```python
from build123d import *

# Parameters (mm, degrees)
SKETCH4_R          = 3
CUT_EXTRUDE1_DEPTH = 11


with BuildPart() as part:
    # Sweep2: sweep along a path in Sketch1
    with BuildLine(Plane(origin=(0, 0, 0), x_dir=(1, 0, 0), z_dir=(0, 1, 0))) as sweep2_path:
        Line((150, 0), (0, 0))
        Line((0, 0), (-89.223418013, -120.578529093))
    # Sketch2 → Sweep2 (sweep)
    with BuildSketch(Plane(origin=(-89.223418013, 0, 120.578529093), x_dir=(0.803856861, 0, 0.594822787), z_dir=(-0.594822787, 0, 0.803856861))):
        Polygon((2.886751346, -5), (5.773502692, 0), (2.886751346, 5), (-2.886751346, 5), (-5.773502692, 0), (-2.886751346, -5), align=None)
    sweep(path=sweep2_path.line, transition=Transition.RIGHT)

    # Sketch4 → Cut-Extrude1 (cut, through all)
    with BuildSketch(Plane(origin=(0, 5, 0), x_dir=(1, 0, 0), z_dir=(0, 1, 0))):
        with Locations((140, 0)):
            Circle(SKETCH4_R)
    cut_extrude1 = extrude(amount=-CUT_EXTRUDE1_DEPTH, mode=Mode.SUBTRACT)

    # Mirror1: Cut-Extrude1 across plane
    add(cut_extrude1.mirror(Plane(origin=(0, 0, 0), x_dir=(0.450098441, 0, 0.892978943), z_dir=(0.892978943, 0, -0.450098441))), mode=Mode.SUBTRACT)


solid = part.part
```
Work out the finished part from the listing and answer in its coordinate system (mm). A direction names the side the tool comes from. Give positions to 0.01 mm unless a question says otherwise; leave off trailing zeros. Loops run counter-clockwise (first coordinate to the right, second up) from the corner with the lowest first, then second, coordinate; pieces in that order, holes last. Notation, with made-up numbers: M 27,82 L 31,82 A16 cw 31,98 Z; hole C 80.5,75 d10. An arc over 180 degrees is marked long. One line per item, written item: value. Start each with the question number.
1. Which of the six approach directions +Z, -Z, +X, -X, +Y, -Y give full straight-line access (tool end or side, diameter ignored) to faces 1 (the face through (74.688, 2.465, 4.35)), 2 (the face through (-89.29, 0.07, 120.53)), 3 (the face through (74.688, -2.535, 4.31))?
2. Find section B-B (x = 47.5). Give the vertices of the cut face in (y, z).
3. Find section D-D (z = 24). Give the vertices of the cut face in (x, y), and give its area (3 significant figures).
4. Determine the mould class of faces 4 (the face through (142.86, 0.07, -0.9)), 5 (the face through (-42.198, -2.535, 64.274)), 6 (the face through (-7, 5, 12)) for opening direction X: released by +X, released by -X, zero draft, split by the parting line, or undercut.
5. Find the intervals of material crossed by probe 1 along X at (y, z) = (0.5, 0); probe 2 along X at (y, z) = (-1, 0); probe 3 along Z at (x, y) = (140, 2.25), in increasing order.
6. Each of these flat-tipped pins is pushed along its axis until it touches: P1, Ø1.5, axis at x = 35.5, y = 1.5, coming from the +Z side; P2, Ø3, axis at x = -57.5, z = 84.5, coming from the +Y side; P3, Ø1.5, axis at x = -12.5, y = -1, coming from the -Z side; P4, Ø2, axis at x = -67.5, y = -4, coming from the -Z side. Where does it stop, or does it pass through?
7. Find section A-A (y = -1.75). Give the vertices of the cut face in (x, z), and give its area (3 significant figures).
8. Find section C-C (z = 0). Give the vertices of the cut face in (x, y), and give its area (3 significant figures).
Reported:
1. face 1: +Z, +X, +Y
1. face 2: +Z, -X, +Y, -Y
1. face 3: +Z, +X, -Y
2. outline: M -5,-2.89 L 0,-5.77 L 5,-2.89 L 5,2.89 L 0,5.77 L -5,2.89 Z
3. outline: M -24.94,0 L -21.35,-5 L -14.17,-5 L -10.58,0 L -14.17,5 L -21.35,5 Z
3. area: 108 mm²
4. face 4: undercut
4. face 5: released by +X
4. face 6: zero draft
5. probe 1: x = -6.82 to 137, 143 to 150
5. probe 2: x = -6.46 to 137, 143 to 150
5. probe 3: z = -4.47 to -3, 3 to 4.47
6. P1: stops at z = 5.34
6. P2: stops at y = 5
6. P3: stops at z = 6.91
6. P4: stops at z = 83.73
7. outline: M -93.05,117.75 L -2.4,-4.76 L 150,-4.76 L 150,4.76 L 2.4,4.76 L -85.39,123.41 Z; hole C -83.28,112.54 d6; hole C 140,0 d6
7. area: 2,800 mm²
8. outline: M -7.18,0 L -3.59,-5 L 137,-5 L 137,5 L -3.59,5 Z; M 143,-5 L 150,-5 L 150,5 L 143,5 Z
8. area: 1,490 mm²
